```python
from build123d import *

# Parameters (mm, degrees)
F1_DEPTH = 60
F2_R     = 1.5
F3_DEPTH = 25
F4_R     = 2.5
F5_R     = 2.5
F6_DEPTH = 5


with BuildPart() as f1:
    # F0 (on Top) → F1 (new body)
    with BuildSketch(Plane.XY):
        with BuildLine():
            Line((-0.8, -20.2), (-0.8, -19.2))
            Line((-0.8, -19.2), (-0.8, -18.500001))
            ThreePointArc((-0.8, -18.500001), (-0.712132, -18.287869), (-0.5, -18.200001))
            Line((-0.5, -18.200001), (1.669121, -18.2))
            ThreePointArc((1.669121, -18.2), (2.389747, -17.718493), (2.220664, -16.868457))
            Line((2.220664, -16.868457), (-0.119113, -14.52868))
            ThreePointArc((-0.119113, -14.52868), (-1.092383, -13.878361), (-2.240433, -13.65))
            Line((-2.240433, -13.65), (-4.509567, -13.65))
            ThreePointArc((-4.509567, -13.65), (-5.657617, -13.878361), (-6.630887, -14.52868))
            Line((-6.630887, -14.52868), (-8.970664, -16.868457))
            ThreePointArc((-8.970664, -16.868457), (-9.139747, -17.718493), (-8.419121, -18.2))
            Line((-8.419121, -18.2), (-6.25, -18.200001))
            ThreePointArc((-6.25, -18.200001), (-6.037868, -18.287869), (-5.95, -18.500001))
            Line((-5.95, -18.500001), (-5.95, -19.2))
            Line((-5.95, -19.2), (-5.95, -20.2))
            Line((-5.95, -20.2), (-8.375, -20.2))
            Line((-8.375, -20.2), (-8.375, -25.2))
            Line((-8.375, -25.2), (-3.375, -25.2))
            Line((-3.375, -25.2), (1.625, -25.2))
            Line((1.625, -25.2), (1.625, -20.2))
            Line((1.625, -20.2), (-0.8, -20.2))
        make_face()
    extrude(amount=-F1_DEPTH)

    # F2 (on face) → F3 (cut)
    with BuildSketch(Plane.XZ.offset(25.2)):
        with Locations((-3.375, -50)):
            Circle(F2_R)
        with Locations((-3.375, -30)):
            Circle(F2_R)
        with Locations((-3.375, -10)):
            Circle(F2_R)
    extrude(amount=-F3_DEPTH, mode=Mode.SUBTRACT)

    # F4 (on face) + F5 (on face) → F6 (cut)
    with BuildSketch(Plane(origin=(0, -13.65, 0), x_dir=(-1, 0, 0), z_dir=(0, 1, 0))):
        with Locations((3.375, -10)):
            Circle(F4_R)
        with Locations((3.375, -30)):
            Circle(F4_R)
    with BuildSketch(Plane(origin=(0, -13.65, 0), x_dir=(-1, 0, 0), z_dir=(0, 1, 0))):
        with Locations((3.375, -50)):
            Circle(F5_R)
    extrude(amount=-F6_DEPTH, mode=Mode.SUBTRACT)


solid = f1.part
```
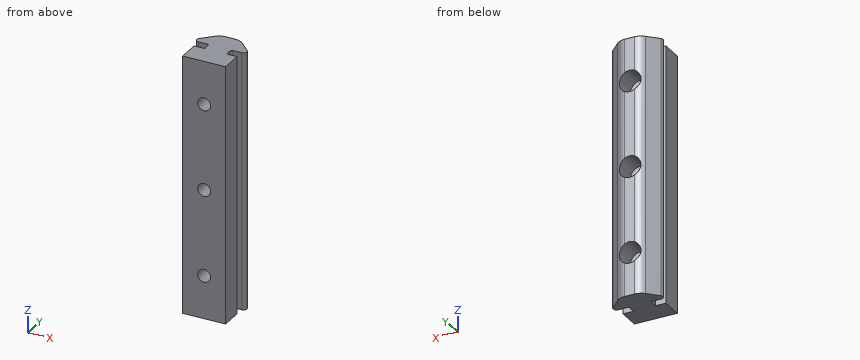
Read the model definition and answer for the solid it produces. Units are mm, in the model's axes. Round coordinates to 2 decimals unless told otherwise and drop trailing zeros. Write each loop counter-clockwise with the first axis right and the second up, starting at its lowest first coordinate (ties: lowest second). Pieces come first, ordered by that corner, then holes. Notation, with made-up numbers: M -8.75,-30.5 L 21.25,-30.5 A29 cw 21.25,-0.5 Z; hole C 31.25,-15.5 d4. An arc over 180 degrees is marked long. One line per item, written item: value.
Q1. Find section A-A on y = -19.25. Write down the section's boundary in (x, z) (3 decimals).
Data:
outline: M -5.95,-60 L -0.8,-60 L -0.8,0 L -5.95,0 Z; hole C -3.375,-50 d3; hole C -3.375,-30 d3; hole C -3.375,-10 d3
Q2. Flat-ended cylindrical pins translate along their axes: pin 1 Ø1.9 at (x, z) = (0.5, -42) entering from +Y; pin 2 Ø2.5 at (y, z) = (-22, -34) entering from -X (3 decimals); pin 3 Ø1.8 at (x, z) = (-3.375, -10) entering from +Y; pin 4 Ø0.5 at (y, z) = (-19.5, -21.5) entering from -X. Find the tip coordinate at first contact, or state that the pin passes through.
Data:
pin 1: y = -14.24
pin 2: x = -8.375
pin 3: through
pin 4: x = -5.95
Q3. Find section C-C on z = -53.5. Write down the section's boundary in (x, y) (3 decimals).
Data:
outline: M -8.971,-16.868 A0.78 ccw -8.419,-18.2 L -6.25,-18.2 A0.3 cw -5.95,-18.5 L -5.95,-20.2 L -8.375,-20.2 L -8.375,-25.2 L 1.625,-25.2 L 1.625,-20.2 L -0.8,-20.2 L -0.8,-18.5 A0.3 cw -0.5,-18.2 L 1.669,-18.2 A0.78 ccw 2.221,-16.868 L -0.119,-14.529 A3 ccw -2.24,-13.65 L -4.51,-13.65 A3 ccw -6.631,-14.529 Z
Q4. Find section B-B on z = -10. Write down the section's boundary in (x, y) (3 decimals), plus the area to 3 significant figures.
Data:
outline: M -8.971,-16.868 A0.78 ccw -8.419,-18.2 L -6.25,-18.2 A0.3 cw -5.95,-18.5 L -5.95,-20.2 L -8.375,-20.2 L -8.375,-25.2 L -4.875,-25.2 L -4.875,-18.65 L -5.875,-18.65 L -5.875,-13.979 A3 ccw -6.631,-14.529 Z; M -1.875,-25.2 L 1.625,-25.2 L 1.625,-20.2 L -0.8,-20.2 L -0.8,-18.5 A0.3 cw -0.5,-18.2 L 1.669,-18.2 A0.78 ccw 2.221,-16.868 L -0.119,-14.529 A3 ccw -0.875,-13.979 L -0.875,-18.65 L -1.875,-18.65 Z
area: 56.4 mm2
Q5. Straight lines are drawn through the part: line 1 (Z direction, x = -3.25, y = -21.75); line 2 (Z direction, x = -5.5, y = -14.5); line 3 (X direction, y = -19.25, z = -35). For each, find the intervals that lie inside material, in ascending order. Write a range as [from, to].
Data:
line 1: [-60, -51.49], [-48.51, -31.49], [-28.51, -11.49], [-8.51, 0]
line 2: [-60, -51.32], [-48.68, -31.32], [-28.68, -11.32], [-8.68, 0]
line 3: [-5.95, -0.8]
Q6. Find section D-D on y = -22.5. Write down the section's boundary in (x, z) (3 decimals).
Data:
outline: M -8.375,-60 L 1.625,-60 L 1.625,0 L -8.375,0 Z; hole C -3.375,-50 d3; hole C -3.375,-30 d3; hole C -3.375,-10 d3
